Read the model definition and answer for the solid it produces. Units are mm, in the model's axes. A direction names the side the tool comes from. Coordinates: 2 decimals unless noted, no trailing zeros. Write each loop counter-clockwise with the first axis right and the second up, starting at its lowest first coordinate (ties: lowest second). Pieces come first, ordered by that corner, then holes. Notation, with made-up numbers: (27, -34) - (44, -34) arc R18 ccw to (44, -6) - close; hole circle Ø10 at (25, -5.5). An arc over 180 degrees is marked (long way). Return JSON: item names as keys, results as strings.
```python
from build123d import *

# Parameters (mm, degrees)
F0_W     = 37.75
F0_H     = 36.75
F1_DEPTH = 15
F3_DEPTH = 14
F4_W     = 7
F4_H     = 14
F5_DEPTH = 5
F6_W     = 10
F6_H     = 14
F7_DEPTH = 3


with BuildPart() as f1:
    # F0 (on Top) → F1 (new body)
    with BuildSketch(Plane.XY):
        with Locations((8.636272, 5.505883)):
            Rectangle(F0_W, F0_H)
    extrude(amount=F1_DEPTH)

    # F2 (on face) → F3 (cut)
    with BuildSketch(Plane(origin=(0, 0, 0), x_dir=(1, 0, 0), z_dir=(0, 0, -1))):
        Polygon((-9.738728, -23.380883), (27.011272, -23.380883), (27.011272, 5.682816), (27.011272, 8.965187), (27.011272, 12.369117), (-9.738728, 12.369117), (-9.738728, -10.72904), (-9.738728, -14.316749), align=None)
    extrude(amount=-F3_DEPTH, mode=Mode.SUBTRACT)

    # F4 (on face) → F5 (cut)
    with BuildSketch(Plane.YZ.offset(27.511272)):
        with Locations((11.380883, 7)):
            Rectangle(F4_W, F4_H)
    extrude(amount=-F5_DEPTH, mode=Mode.SUBTRACT)

    # F6 (on face) → F7 (cut)
    with BuildSketch(Plane(origin=(-10.238728, 0, 0), x_dir=(0, -1, 0), z_dir=(-1, 0, 0))):
        with Locations((-2.880883, 7)):
            Rectangle(F6_W, F6_H)
    extrude(amount=-F7_DEPTH, mode=Mode.SUBTRACT)


solid = f1.part
```
(1) Which of the six approach directions +Z, -Z, +X, -X, +Y, -Y give full straight-line access (tool end or side, diameter ignored) to faces 1 (the face through (27.011, 19, 7)), 2 (the face through (27.511, 5, 7))?
Answer:
{"face 1": "-Z", "face 2": "+Z, -Z, +X, +Y, -Y"}
(2) Determine the mould class of faces 3 (the face through (8, 6, 14)), 4 (the face through (8, 23.881, 7)), 5 (the face through (-10.239, 9, 7)) for opening direction X: +X half, -X half, draft (parallel to the pull), parting line (faces both ways), or undercut.
Answer:
{"face 3": "undercut", "face 4": "draft", "face 5": "-X half"}
(3) A cutting plane is placed at B-B (x = 2). Determine the outline of the cut face in (y, z).
Answer:
{"outline": "(-12.87, 0) - (-12.37, 0) - (-12.37, 14) - (23.38, 14) - (23.38, 0) - (23.88, 0) - (23.88, 15) - (-12.87, 15) - close"}
(4) Straight lines are drawn through the part: line 1 (Y direction, x = 13.5, z = 8); line 2 (X direction, y = -6, z = 1); line 3 (Z direction, x = -5.5, y = 8). For each, find the intervals that lie inside material, in ascending order. Write a range as from..to.
Answer:
{"line 1": "-12.87..-12.37, 23.38..23.88", "line 2": "-10.24..-9.74, 27.01..27.51", "line 3": "14..15"}
(5) A cutting plane is placed at C-C (y = -5). Determine the outline of the cut face in (x, z), and give its area (4 significant figures).
Answer:
{"outline": "(-10.24, 0) - (-9.74, 0) - (-9.74, 14) - (27.01, 14) - (27.01, 0) - (27.51, 0) - (27.51, 15) - (-10.24, 15) - close", "area": "51.75 mm²"}
(6) A cutting plane is placed at D-D (y = 12). Determine the outline of the cut face in (x, z), and give its area (4 significant figures).
Answer:
{"outline": "(-10.24, 0) - (-9.74, 0) - (-9.74, 14) - (27.51, 14) - (27.51, 15) - (-10.24, 15) - close", "area": "44.75 mm²"}
(7) A cutting plane is placed at A-A (z = 7.5). Determine the outline of the cut face in (x, y).
Answer:
{"outline": "(-10.24, -12.87) - (27.51, -12.87) - (27.51, 7.88) - (27.01, 7.88) - (27.01, -12.37) - (-9.74, -12.37) - (-9.74, -2.12) - (-10.24, -2.12) - close; (-10.24, 7.88) - (-9.74, 7.88) - (-9.74, 23.38) - (27.01, 23.38) - (27.01, 14.88) - (27.51, 14.88) - (27.51, 23.88) - (-10.24, 23.88) - close"}
(8) A flat-ended cylindrical pin translates along its axis: P1, Ø18, axis at x = 17, y = 5.5, coming from the -Z side. Find the tip coordinate at first contact, or state that the pin passes through.
Answer:
{"P1": "z = 14"}
